```python
from build123d import *

# Parameters (mm, degrees)
EXTRUDE_1_DEPTH          = 300
CUT_EXTRUDE_1_DEPTH      = 1.0000001
CUT_EXTRUDE_1_DEPTH_BACK = 831.0000001
SKETCH_4_W               = 15
SKETCH_4_H               = 45
CUT_EXTRUDE_2_DEPTH      = 258.720162759
SKETCH_4_3_W             = 15
SKETCH_4_3_H             = 45
CUT_EXTRUDE_3_DEPTH      = 20


with BuildPart() as part:
    # 스케치1 → 보스-돌출1 (new body)
    with BuildSketch(Plane(origin=(0, 0, 0), x_dir=(0, 0, -1), z_dir=(1, 0, 0))):
        with BuildLine():
            Line((-41.993007726, 32.892860384), (-41.993007726, -303.619075042))
            Line((-41.993007726, -303.619075042), (788.006992274, -303.619075042))
            Line((788.006992274, -303.619075042), (788.006992274, -12.90547458))
            add(Edge.make_bspline(
                [(788.006992274, -12.90547458), (680.261509472, 78.254339674), (631.210016853, 128.415858034), (368.750142796, 135.255878696)],
                knots=[0, 0, 0, 0, 1, 1, 1, 1], degree=3))
            add(Edge.make_bspline(
                [(45.325655749, 132.198658827), (134.989620851, 137.211386353), (265.463569923, 138.011524869), (368.750142796, 135.255878696)],
                knots=[0, 0, 0, 0, 1, 1, 1, 1], degree=3))
            Line((45.325655749, 132.198658827), (-41.993007726, 32.892860384))
        make_face()
        with BuildLine():
            Line((4.116595834, 54.214584045), (54.427658026, 114.389853292))
            add(Edge.make_bspline(
                [(54.427658026, 114.389853292), (122.914694658, 118.068796405), (254.727094278, 116.434615788), (344.321994749, 115.599177573)],
                knots=[0, 0, 0, 0, 0.843637698, 0.843637698, 0.843637698, 0.843637698], degree=3))
            Line((344.321994749, 115.599177573), (359.116595834, -53.619075042))
            Line((359.116595834, -53.619075042), (4.116595834, -53.619075042))
            Line((4.116595834, -53.619075042), (4.116595834, 54.214584045))
        make_face(mode=Mode.SUBTRACT)
        with BuildLine():
            Line((414.932922958, -53.619075042), (389.116595834, 115.255878696))
            add(Edge.make_bspline(
                [(389.116595834, 115.255878696), (584.597474826, 110.825479528), (668.447748965, 84.913988672), (744.116595834, 1.380924958)],
                knots=[0.027735734, 0.027735734, 0.027735734, 0.027735734, 0.842070206, 0.842070206, 0.842070206, 0.842070206], degree=3))
            Line((744.116595834, 1.380924958), (744.116595834, -53.619075042))
            Line((744.116595834, -53.619075042), (414.932922958, -53.619075042))
        make_face(mode=Mode.SUBTRACT)
    extrude(amount=EXTRUDE_1_DEPTH)

    # 스케치2 → 컷-돌출1 (cut, two sides)
    with BuildSketch(Plane.XY.offset(41.993007726)) as cut_extrude_1_sk:
        Polygon((179.652203691, 32.892860384), (239.655287588, 136.821250303), (282.956557777, 111.821250303), (237.38723061, 32.892860384), (300, 32.892860384), (300, -303.619075042), (341.364714008, -303.619075042), (341.364714008, 251.457374482), (0, 251.457374482), (0, 32.892860384), align=None)
        Polygon((95.31772029, -113.178749697), (179.652203691, 32.892860384), (0, 32.892860384), (0, -303.619075042), (95.31772029, -303.619075042), align=None)
        Polygon((300, 32.892860384), (237.38723061, 32.892860384), (153.052747209, -113.178749697), (153.052747209, -303.619075042), (300, -303.619075042), align=None)
    extrude(amount=CUT_EXTRUDE_1_DEPTH, mode=Mode.SUBTRACT)
    extrude(cut_extrude_1_sk.sketch, amount=-CUT_EXTRUDE_1_DEPTH_BACK, mode=Mode.SUBTRACT)

    # 스케치4 → 컷-돌출2 (cut, through all)
    with BuildSketch(Plane(origin=(120.496126421, -69.568471025, 0), x_dir=(0, 0, 1), z_dir=(-0.866025404, 0.5, 0))):
        with Locations((-374.116595834, 175.489898801)):
            Rectangle(SKETCH_4_W, SKETCH_4_H)
    extrude(amount=-CUT_EXTRUDE_2_DEPTH, mode=Mode.SUBTRACT)

    # 스케치4<3> → 컷-돌출3 (cut)
    with BuildSketch(Plane(origin=(120.496126421, -69.568471025, 0), x_dir=(0, 0, 1), z_dir=(-0.866025404, 0.5, 0))):
        Polygon((-744.116595834, 18.416776129), (-744.116595834, 213.416776129), (-389.116595834, 213.416776129), (-389.116595834, 17.989898801), (-389.116595834, -11.583223871), (-744.116595834, -11.583223871), align=None)
        Polygon((-359.116595834, 18.416776129), (-359.116595834, 212.989898801), (-4.116595834, 212.989898801), (-4.116595834, 17.989898801), (-4.116595834, -12.010101199), (-359.116595834, -12.010101199), align=None)
        with Locations((-374.116595834, 175.489898801)):
            Rectangle(SKETCH_4_3_W, SKETCH_4_3_H)
    extrude(amount=-CUT_EXTRUDE_3_DEPTH, mode=Mode.SUBTRACT)


solid = part.part
```
CAD build for the part. Positions are in the model's coordinates, mm. A direction names the side the tool comes from. Round coordinates to 2 decimals unless told otherwise and drop trailing zeros. Loops run counter-clockwise (first coordinate to the right, second up) from the corner with the lowest first, then second, coordinate; pieces in that order, holes last. Notation, with made-up numbers: (46, -29) - (92, -29) arc R35 ccw to (92, 10) - close; hole circle Ø10 at (-20.75, 32). An arc over 180 degrees is marked (long way). Return JSON: item names as keys, results as strings. Group by question number.
Q1. Two-plate mould, pull along X, no slides. Class faces 1 (the face through (229, 70, -381.617)), 2 (the face through (123.24, -84.53, -564.13)), 3 (the face through (151.038, -56.669, -539.492)), 4 (the face through (235.53, 109.956, -351.854)): +X half, -X half, draft (parallel to the pull), parting line (faces both ways), or undercut.
Q2. Flat gauge pins, fed straight in: pin 1 Ø19 at (x, y) = (213.5, 59) entering from -Z; pin 2 Ø8 at (x, z) = (131, -300) entering from +Y; pin 3 Ø3 at (x, z) = (173.5, -492) entering from -Y. Where does each tip first touch, or does it go through?
Q3. Tool access for faces 5 (the face through (233.14, 85.54, -20.3)), 6 (the face through (235.53, 109.956, -38.518)), 7 (the face through (248.53, 83.88, -28.92)), 8 (the face through (153.053, -207, -367)): list every direction of +Z, -Z, +X, -X, +Y, -Y with a clear straight run to the whole face (end or side of a thin tool).
Q4. Band-saw the part on A-A on y = -254. Give the cut face in (x, z), plus the area to 3 significant figures.
Q5. Drill centre lines: line 1 along Z through (x, y) = (131.5, -55); line 2 along Z through (x, y) = (189, -42); line 3 along X through (y, z) = (-189, -542.5). Where is each one in solid material? Low to high. Write a range as [from, to].
Solutions:
{
 "1": {"face 1": "draft", "face 2": "undercut", "face 3": "undercut", "face 4": "-X half"},
 "2": {"pin 1": "stops at z = -711.56", "pin 2": "stops at y = -84.45", "pin 3": "stops at y = -80.36"},
 "3": {"face 5": "-X", "face 6": "+Z, -X", "face 7": "+X, -X, -Y", "face 8": "+Z, -Z, +X, -Y"},
 "4": {"outline": "(95.32, -788.01) - (153.05, -788.01) - (153.05, 41.99) - (95.32, 41.99) - close", "area": "47,900 mm^2"},
 "5": {"line 1": "z = [-788.01, -744.12], [-389.12, -359.12], [-4.12, 41.99]", "line 2": "z = [-788.01, -744.12], [-413.16, -358.1], [-4.12, 41.99]", "line 3": "x = [95.32, 153.05]"}
}
